Here's the drawing with two shaded views (mm, measured from the low corner). I have some questions. A direction names the side the tool comes from. Give positions to 0.01 mm unless a question says otherwise; leave off trailing zeros. Loops run counter-clockwise (first coordinate to the right, second up) from the corner with the lowest first, then second, coordinate; pieces in that order, holes last.
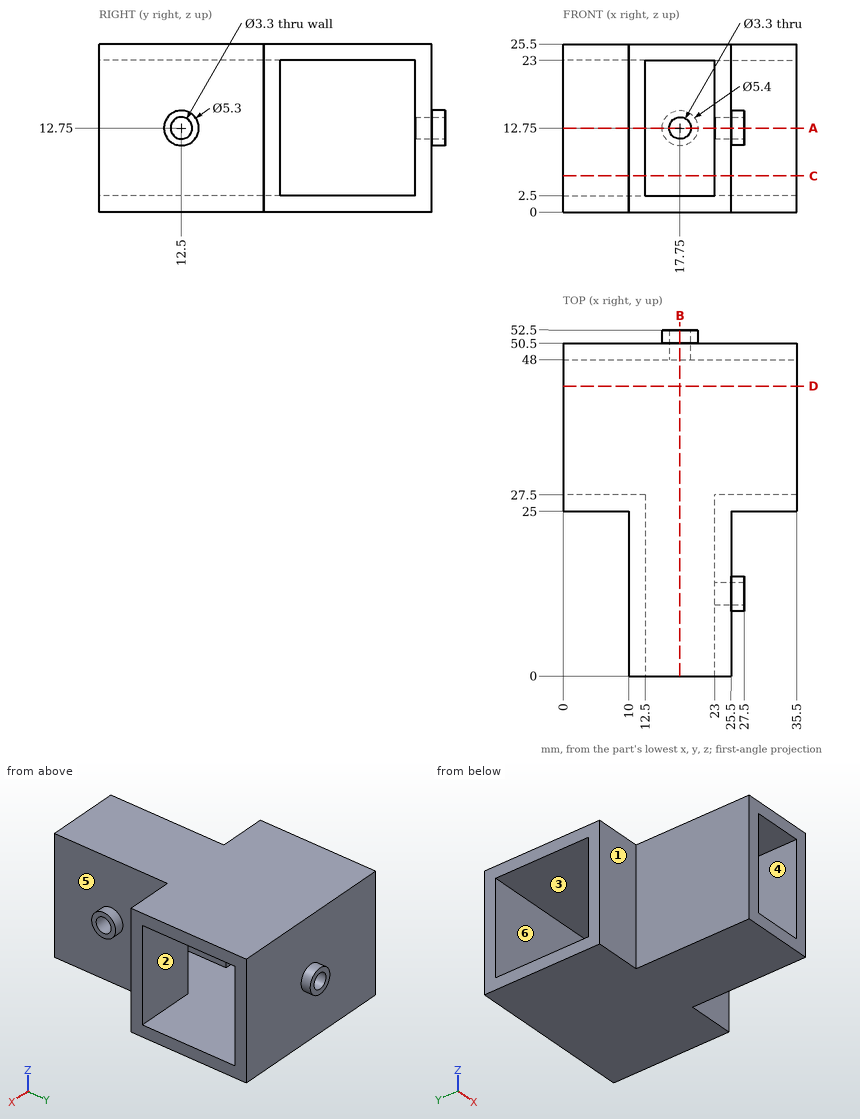
(1) Please list where these lines run through material, in increasing order: probe 1 along Y at (x, z) = (34.5, 18.5); probe 2 along Z at (x, y) = (25.65, 12.5); probe 3 along X at (y, z) = (23, 17.75).
Returned:
probe 1: y = 25 to 27.5, 48 to 50.5
probe 2: z = 10.1 to 11.1, 14.4 to 15.4
probe 3: x = 10 to 12.5, 23 to 25.5
(2) Suppose I cut it at C-C on z = 5.5. List the corners of the cut face in (x, y) for me.
Returned:
outline: (0, 25) - (10, 25) - (10, 0) - (12.5, 0) - (12.5, 27.5) - (0, 27.5) - close; (0, 48) - (35.5, 48) - (35.5, 50.5) - (0, 50.5) - close; (23, 0) - (25.5, 0) - (25.5, 25) - (35.5, 25) - (35.5, 27.5) - (23, 27.5) - close
(3) Thinking about a two-plate mould opening in X: for the marked faces 4, 5 and 6, which applies, pulls with the +X half, pulls with the -X half, needs draft (parallel to the pull), parting line crosses it, or undercut?
Returned:
face 4: undercut
face 5: pulls with the +X half
face 6: needs draft
(4) Which directions (+Z, -Z, +X, -X, +Y, -Y) give clear straight access to the entire face, cutting with the end or side of a thin tool? Please do the marked faces 1, 2 and 3.
Returned:
face 1: +Z, -Z, -X, -Y
face 2: +X, -X
face 3: none
(5) Suppose I cut it at A-A on z = 12.75. Give the number of separate pieces and of enclosed holes in the cut face, plus the area to 3 significant figures.
Returned:
separate pieces: 5
enclosed holes: 0
area: 268 mm2
(6) Suppose I cut it at D-D on y = 44. List the corners of the cut face in (x, z) for me, plus the area to 4 significant figures.
Returned:
outline: (0, 0) - (35.5, 0) - (35.5, 2.5) - (0, 2.5) - close; (0, 23) - (35.5, 23) - (35.5, 25.5) - (0, 25.5) - close
area: 177.5 mm2
(7) Will these pins go through, and if not, where does the flat tip stop? P1, Ø5, axis at x = 7, z = 6.5, coming from the -Y side; P2, Ø5, axis at y = 21, z = 19.5, coming from the +X side; P3, Ø12, axis at y = 9, z = 14, coming from the -X side; P4, Ø2.5, axis at x = 17.75, z = 12.75, coming from the -Y side.
Returned:
P1: stops at y = 25
P2: stops at x = 25.5
P3: stops at x = 10
P4: passes through
(8) Suppose I cut it at B-B on x = 17.75. List the corners of the cut face in (y, z) for me.
Returned:
outline: (0, 0) - (50.5, 0) - (50.5, 10.05) - (52.5, 10.05) - (52.5, 11.1) - (48, 11.1) - (48, 2.5) - (0, 2.5) - close; (0, 23) - (48, 23) - (48, 14.4) - (52.5, 14.4) - (52.5, 15.45) - (50.5, 15.45) - (50.5, 25.5) - (0, 25.5) - close
